```python
from build123d import *

# Parameters (mm, degrees)
SKETCH1_W           = 6.873579398
SKETCH1_H           = 7.9375
BOSS_EXTRUDE1_DEPTH = 1
SKETCH2_W           = 6.35
SKETCH2_H           = 6.35
BOSS_EXTRUDE2_DEPTH = 10


with BuildPart() as part:
    # Sketch1 → Boss-Extrude1 (new body)
    with BuildSketch(Plane(origin=(0, 0, 0), x_dir=(1, 0, 0), z_dir=(0, 1, 0))):
        Rectangle(SKETCH1_W, SKETCH1_H)
        with BuildLine():
            ThreePointArc((3.436789699, 3.96875), (0, 5.25), (-3.436789699, 3.96875))
            Line((-3.436789699, 3.96875), (3.436789699, 3.96875))
        make_face()
        with BuildLine():
            Line((3.436789699, -3.96875), (-3.436789699, -3.96875))
            ThreePointArc((-3.436789699, -3.96875), (0, -5.25), (3.436789699, -3.96875))
        make_face()
    extrude(amount=BOSS_EXTRUDE1_DEPTH)

    # Sketch2 → Boss-Extrude2 (add)
    with BuildSketch(Plane(origin=(0, 1, 0), x_dir=(1, 0, 0), z_dir=(0, 1, 0))):
        with BuildLine():
            Line((-3.436789699, 3.96875), (-3.436789699, -3.96875))
            ThreePointArc((-3.436789699, -3.96875), (0, -5.25), (3.436789699, -3.96875))
            Line((3.436789699, -3.96875), (3.436789699, 3.96875))
            ThreePointArc((3.436789699, 3.96875), (0, 5.25), (-3.436789699, 3.96875))
        make_face()
        Rectangle(SKETCH2_W, SKETCH2_H, mode=Mode.SUBTRACT)
    extrude(amount=BOSS_EXTRUDE2_DEPTH)


solid = part.part
```
Could you check a few things on this model? Use its own coordinates, in mm. A direction names the side the tool comes from. Coordinates: 2 decimals unless noted, no trailing zeros. Write each loop counter-clockwise with the first axis right and the second up, starting at its lowest first coordinate (ties: lowest second). Pieces come first, ordered by that corner, then holes. Notation, with made-up numbers: (45, 16.5) -> (86, 16.5) arc R14 ccw to (86, 39.5) -> close; hole circle Ø8 at (70, 64.25). An arc over 180 degrees is marked (long way). Write item = value, one per line. Start each with the question number.
(1) Will this pin go through, and if not, where does the flat tip stop? pin 1 (3 mm diameter, centred on x = -1.5, z = -1.5, fed in from +Y).
(2) I need wall thicknesses on line 1 (X direction, y = 8.75, z = -0.25) (3 decimals); line 2 (Y direction, x = -3, z = -1.5); line 3 (Z direction, x = -2.25, y = 2.5) (3 decimals). Which ranges of each line are inside material? Lowest first, please. Write a range as [from, to].
(3) Which directions (+Z, -Z, +X, -X, +Y, -Y) give clear straight access to the entire face, cutting with the end or side of a thin tool? Please do faces 4 (the face through (-3.437, 5, 0)), 5 (the face through (0, 6, 3.175)).
(4) I want a section at B-B (y = 4.75). Please give me the cut outline in (x, z) (3 decimals).
(5) We'd pull the mould along X, two halves only. Please class faces 1 (the face through (3.175, 6, 0)), 2 (the face through (3.437, 5, 0)), 3 (the face through (-0.05, 5.42, 5.25)): released by +X, released by -X, zero draft, split by the parting line, or undercut.
(6) I want a section at A-A (z = 1.5). Please give me the cut outline in (x, y) (3 decimals).
(7) I want a section at C-C (x = 0). Please give me the cut outline in (y, z) (3 decimals), plus the area to 3 significant figures.
Result set:
q1.pin_1 = 1
q2.line_1 = [-3.437, -3.175], [3.175, 3.437]
q2.line_2 = [0, 1]
q2.line_3 = [-4.743, -3.175], [3.175, 4.743]
q3.face_4 = +Z, -Z, -X, +Y, -Y
q3.face_5 = +Y
q4.outline = (-3.437, -3.969) arc R5.25 ccw to (3.437, -3.969) -> (3.437, 3.969) arc R5.25 ccw to (-3.437, 3.969) -> close; hole (-3.175, -3.175) -> (3.175, -3.175) -> (3.175, 3.175) -> (-3.175, 3.175) -> close
q5.face_1 = undercut
q5.face_2 = released by +X
q5.face_3 = split by the parting line
q6.outline = (-3.437, 0) -> (3.437, 0) -> (3.437, 11) -> (3.175, 11) -> (3.175, 1) -> (-3.175, 1) -> (-3.175, 11) -> (-3.437, 11) -> close
q7.outline = (0, -5.25) -> (11, -5.25) -> (11, -3.175) -> (1, -3.175) -> (1, 3.175) -> (11, 3.175) -> (11, 5.25) -> (0, 5.25) -> close
q7.area = 52.0 mm2
